Part model, mm, in its own coordinate system. A direction names the side the tool comes from. Coordinates: 2 decimals unless noted, no trailing zeros. Order: outer loops, then holes, each group sorted by start corner. A loop starts at its lowest first (then second) coordinate and runs counter-clockwise, first axis right, second up. Notation, with made-up numbers: M 68,79.5 L 111,79.5 A18 ccw 111,96.5 Z; hole C 32,-12 d8. An arc over 180 degrees is marked long. Answer in a Markdown table with one row per item. Add a question column.
from build123d import *

# Parameters (mm, degrees)
F0_W     = 88.9
F0_H     = 203.2
F1_DEPTH = 38.1
F2_R     = 6.35
F3_DEPTH = 25.4


with BuildPart() as f1:
    # F0 (on Top) → F1 (new body)
    with BuildSketch(Plane.XY):
        Rectangle(F0_W, F0_H)
    extrude(amount=F1_DEPTH)

    # F2 (on Top) → F3 (join)
    with BuildSketch(Plane.XY):
        Circle(F2_R)
    extrude(amount=-F3_DEPTH)


solid = f1.part
(1) Slice it at A-A (y = 0). List the corners of the cut face in (x, z), and give its area (3 significant figures).
(2) Slice it at D-D (y = -70). List the corners of the cut face in (x, z), and give its area (3 significant figures).
(3) Slice it at B-B (x = 0). List the corners of the cut face in (y, z), and give its area (3 significant figures).
(4) Slice it at C-C (x = -36). List the corners of the cut face in (y, z).
(5) 3-axis set-ups, long thin cutter, end or side, ignore diameter. For faces 1 (the flat face through (-1, 101.6, 19)), 2 (the cylindrical face through (-1.38, -6.2, -12.52)): which of +Z, -Z, +X, -X, +Y, -Y reach the whole face in a straight line?
(6) Wall check: line 1 (Z direction, x = 11, y = -65.5); line 2 (Y direction, x = 4.5, z = -17.5). Give the ranges that are in metal, low to high.
(7) Drop a flat-ended pin along its axis: P1, Ø1, axis at x = -4.5, y = -18, coming from the -Z side. Give the stop position or say it passes through.
Computed:
| question | item | result |
|---|---|---|
| 1 | outline | M -44.45,0 L -6.35,0 L -6.35,-25.4 L 6.35,-25.4 L 6.35,0 L 44.45,0 L 44.45,38.1 L -44.45,38.1 Z |
| 1 | area | 3,710 mm^2 |
| 2 | outline | M -44.45,0 L 44.45,0 L 44.45,38.1 L -44.45,38.1 Z |
| 2 | area | 3,390 mm^2 |
| 3 | outline | M -101.6,0 L -6.35,0 L -6.35,-25.4 L 6.35,-25.4 L 6.35,0 L 101.6,0 L 101.6,38.1 L -101.6,38.1 Z |
| 3 | area | 8,060 mm^2 |
| 4 | outline | M -101.6,0 L 101.6,0 L 101.6,38.1 L -101.6,38.1 Z |
| 5 | face 1 | +Z, -Z, +X, -X, +Y |
| 5 | face 2 | -Z |
| 6 | line 1 | z = 0 to 38.1 |
| 6 | line 2 | y = -4.48 to 4.48 |
| 7 | P1 | stops at z = 0 |
